Part print with two shaded views. Sizes in mm from the minimum x, y, z corner. Coordinates: 2 decimals unless noted, no trailing zeros. Loops run counter-clockwise (first coordinate to the right, second up) from the corner with the lowest first, then second, coordinate; pieces in that order, holes last.
Item 1: Cut at B-B (x = 60.5). List the corners of the cut face in (y, z).
Item 2: Cut at C-C (z = 1.2). List the corners of the cut face in (x, y).
Item 3: Cut at A-A (y = 6). List the corners of the cut face in (x, z) (1 decimal).
Item 4: Drill centre lines: line 1 along X through (y, z) = (42, 2.75) (1 decimal); line 2 along Y through (x, z) = (43, 4.35) (1 decimal); line 3 along Y through (x, z) = (52, 1.7) (1 decimal). Where is each one in solid material? Low to high.
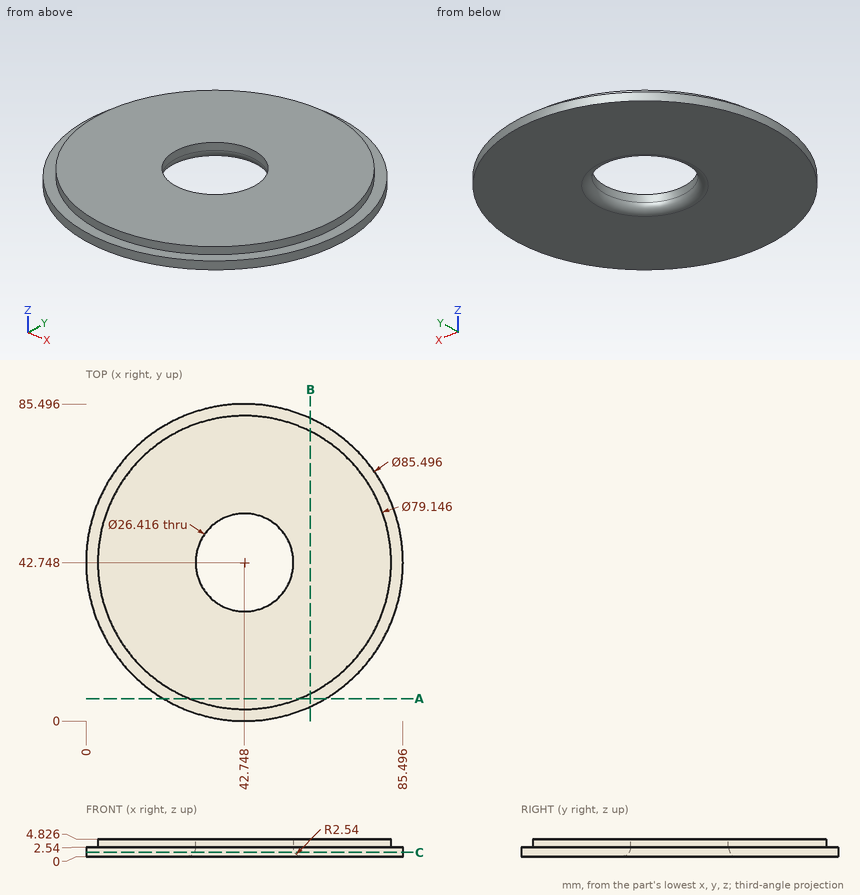
Filled sheet:
1. outline: (3.86, 0) - (81.64, 0) - (81.64, 2.54) - (78.12, 2.54) - (78.12, 4.83) - (7.38, 4.83) - (7.38, 2.54) - (3.86, 2.54) - close
2. outline: circle Ø85.5 at (42.75, 42.75); hole circle Ø27.18 at (42.75, 42.75)
3. outline: (20.9, 0) - (64.6, 0) - (64.6, 2.5) - (57.4, 2.5) - (57.4, 4.8) - (28.1, 4.8) - (28.1, 2.5) - (20.9, 2.5) - close
4. line 1: x = 3.2 to 29.6, 55.9 to 82.3
4. line 2: y = 3.2 to 29.5, 56 to 82.3
4. line 3: y = 1 to 33.1, 52.4 to 84.5
